The listing builds one solid part. Answer for the finished solid, in the listing's coordinates (mm). A direction names the side the tool comes from. Give positions to 0.01 mm unless a question says otherwise; leave off trailing zeros. Loops run counter-clockwise (first coordinate to the right, second up) from the corner with the lowest first, then second, coordinate; pieces in that order, holes last. Notation, with made-up numbers: (-10.5, 37.25) - (34.5, 37.25) arc R24 ccw to (34.5, 71.25) - close; hole circle Ø8 at (1.25, 13.25). An arc over 180 degrees is marked (long way). Write item = value, one per line. Start each with the question number.
1) The part is cut by section A-A on x = 19.05. Write down the section's boundary in (y, z) (3 decimals), plus the area to 3 significant figures.
2) The mould has two halves that part along Y. Classify faces 1 (the flat face through (69, -3.175, 2)), 2 (the cylindrical face through (16.1, -10.7, 1.6)), 3 (the flat face through (64.77, -17, 2)): +Y half, -Y half, draft (parallel to the pull), parting line (faces both ways), or undercut.
3) Flat-ended cylindrical pins translate along their axes: P1, Ø1, axis at y = -1.5, z = 1.5, coming from the -X side; P2, Ø1, axis at x = 37.5, z = 2, coming from the -Y side (3 decimals); P3, Ø1, axis at y = -17, z = 2, coming from the +X side. Find the tip coordinate at first contact, or state that the pin passes through.
4) The part is cut by section C-C on z = 0.9. Write down the section's boundary in (x, y) (3 decimals), plus the area to 3 significant figures.
5) Which of the six approach directions +Z, -Z, +X, -X, +Y, -Y give full straight-line access (tool end or side, diameter ignored) to faces 4 (the flat face through (11.43, -2, 2)), 5 (the flat face through (38, -3.175, 2)), 6 (the flat face through (46.99, -17, 2))?
6) The part is cut by section D-D on x = 37.5. Write down the section's boundary in (y, z) (3 decimals), plus the area to 3 significant figures.
7) Consider probe 1 along X at (y, z) = (-16, 0.45); probe 2 along X at (y, z) = (-10, 1.3); probe 3 along Y at (x, z) = (57.15, 0.8). Determine where each line is inside the solid, lowest interval first.
8) The part is cut by section B-B on y = -8.25. Write down the section's boundary in (x, z) (3 decimals).
from build123d import *

# Parameters (mm, degrees)
SKETCH1_W               = 76.2
SKETCH1_H               = 19.05
BOSS_EXTRUDE1_DEPTH     = 3.175
SKETCH2_W               = 11.43
SKETCH2_H               = 3.175
CUT_EXTRUDE1_DEPTH      = 79.60930686
SKETCH3_W               = 17.78
SKETCH3_H               = 3.175
CUT_EXTRUDE2_DEPTH      = 79.60930686
MIRROR2_COPY_1_SKETCH_W = 11.43
MIRROR2_COPY_1_SKETCH_H = 3.175
MIRROR2_COPY_1_DEPTH    = 79.60930686
HOLE1_D                 = 6.35
SKETCH6_W               = 3.175
SKETCH6_H               = 12.7
CUT_EXTRUDE3_DEPTH      = 3.81
SKETCH7_W               = 3.175
SKETCH7_H               = 12.7
CUT_EXTRUDE4_DEPTH      = 3.81


with BuildPart() as part:
    # Sketch1 → Boss-Extrude1 (new body)
    with BuildSketch(Plane.XY):
        with Locations((38.1, -9.525)):
            Rectangle(SKETCH1_W, SKETCH1_H)
    extrude(amount=BOSS_EXTRUDE1_DEPTH)

    # Sketch2 → Cut-Extrude1 (cut, through all)
    with BuildSketch(Plane.XY.offset(3.175)):
        with Locations((5.715, -1.5875)):
            Rectangle(SKETCH2_W, SKETCH2_H)
    cut_extrude1 = extrude(amount=-CUT_EXTRUDE1_DEPTH, mode=Mode.SUBTRACT)

    # Mirror1: Cut-Extrude1 across plane
    add(cut_extrude1.mirror(Plane(origin=(38.1, 0, 0), x_dir=(0, 0, 1), z_dir=(1, 0, 0))), mode=Mode.SUBTRACT)

    # Sketch3 → Cut-Extrude2 (cut, through all)
    with BuildSketch(Plane.XY.offset(3.175)):
        with Locations((38.1, -1.5875)):
            Rectangle(SKETCH3_W, SKETCH3_H)
    cut_extrude2 = extrude(amount=-CUT_EXTRUDE2_DEPTH, mode=Mode.SUBTRACT)

    # Mirror2: Cut-Extrude1, Cut-Extrude2 across plane
    add(cut_extrude1.mirror(Plane.ZX.offset(-9.525)), mode=Mode.SUBTRACT)
    add(cut_extrude2.mirror(Plane.ZX.offset(-9.525)), mode=Mode.SUBTRACT)

    # Mirror2 copy 1 sketch → Mirror2 copy 1 (cut, through all)
    with BuildSketch(Plane(origin=(76.2, -19.05, 3.175), x_dir=(-1, 0, 0), z_dir=(0, 0, 1))):
        with Locations((5.715, -1.5875)):
            Rectangle(MIRROR2_COPY_1_SKETCH_W, MIRROR2_COPY_1_SKETCH_H)
    extrude(amount=-MIRROR2_COPY_1_DEPTH, mode=Mode.SUBTRACT)

    # Hole1 (through all)
    with Locations(Plane.XY.offset(3.175)):
        with Locations((19.05, -9.525), (57.15, -9.525)):
            Hole(HOLE1_D / 2)

    # Sketch6 → Cut-Extrude3 (cut)
    with BuildSketch(Plane.ZY):
        with Locations((1.5875, -9.525)):
            Rectangle(SKETCH6_W, SKETCH6_H)
    extrude(amount=-CUT_EXTRUDE3_DEPTH, mode=Mode.SUBTRACT)

    # Sketch7 → Cut-Extrude4 (cut)
    with BuildSketch(Plane(origin=(76.2, 0, 0), x_dir=(0, 0, -1), z_dir=(1, 0, 0))):
        with Locations((-1.5875, -9.525)):
            Rectangle(SKETCH7_W, SKETCH7_H)
    extrude(amount=-CUT_EXTRUDE4_DEPTH, mode=Mode.SUBTRACT)


solid = part.part
Answer below:
q1.outline = (-19.05, 0) - (-12.7, 0) - (-12.7, 3.175) - (-19.05, 3.175) - close; (-6.35, 0) - (0, 0) - (0, 3.175) - (-6.35, 3.175) - close
q1.area = 40.3 mm2
q2.face_1 = +Y half
q2.face_2 = undercut
q2.face_3 = draft
q3.P1 = 11.43
q3.P2 = -15.875
q3.P3 = 64.77
q4.outline = (3.81, -15.875) - (11.43, -15.875) - (11.43, -19.05) - (29.21, -19.05) - (29.21, -15.875) - (46.99, -15.875) - (46.99, -19.05) - (64.77, -19.05) - (64.77, -15.875) - (72.39, -15.875) - (72.39, -3.175) - (64.77, -3.175) - (64.77, 0) - (46.99, 0) - (46.99, -3.175) - (29.21, -3.175) - (29.21, 0) - (11.43, 0) - (11.43, -3.175) - (3.81, -3.175) - close; hole circle Ø6.35 at (19.05, -9.525); hole circle Ø6.35 at (57.15, -9.525)
q4.area = 1,030 mm2
q5.face_4 = +Z, -Z, -X, +Y
q5.face_5 = +Z, -Z, +Y
q5.face_6 = +Z, -Z, -Y
q6.outline = (-15.875, 0) - (-3.175, 0) - (-3.175, 3.175) - (-15.875, 3.175) - close
q6.area = 40.3 mm2
q7.probe_1 = 11.43 to 29.21, 46.99 to 64.77
q7.probe_2 = 3.81 to 15.91, 22.19 to 54.01, 60.29 to 72.39
q7.probe_3 = -19.05 to -12.7, -6.35 to 0
q8.outline = (3.81, 0) - (16.142, 0) - (16.142, 3.175) - (3.81, 3.175) - close; (21.958, 0) - (54.242, 0) - (54.242, 3.175) - (21.958, 3.175) - close; (60.058, 0) - (72.39, 0) - (72.39, 3.175) - (60.058, 3.175) - close
